Autodesk Inventor part; units mm, degrees
ref_plane "YZ Plane" through (0, 0, 0) normal (1, 0, 0) x (0, 1, 0)
ref_plane "XZ Plane" through (0, 0, 0) normal (0, 1, 0) x (-1, 0, 0)
ref_plane "XY Plane" through (0, 0, 0) normal (0, 0, 1) x (1, 0, 0)
sketch "スケッチ3" plane through (0, 0, 0) normal (0, 0, 1) x (1, 0, 0)
  line L0 (0, 0) -> (0, 5)
  line L1 (0, 5) -> (-10, 5)
  line L2 (-10, 5) -> (-20, 15)
  line L3 (-20, 15) -> (-35, 15)
  line L4 (-35, 15) -> (-45, 5)
  line L5 (-45, 5) -> (-55, 15)
  line L6 (-80, 0) -> (0, 0)
  line L7 (0, 5) -> (0, 0)
  line L8 (-55, 15) -> (-80, 15)
  line L9 (-80, 15) -> (-80, 0)
  dimension "d0" = 10
  dimension "d2" = 15
  dimension "d4" = 5
  dimension "d6" = 135
  dimension "d9" = 25
  dimension "d10" = 15
extrude "押し出し1" add sketch "スケッチ3" along normal blind 15
chamfer "面取り1" distance 4 angle 45 1 edges at (-80, 15, 7.5)
sketch "スケッチ4" plane through (0, 0, 15) normal (0, 0, 1) x (1, 0, 0)
  line L0 (-80, 11) -> (-76, 15)
  line L1 (-80, 11) -> (-80, 0)
  line L2 (-80, 0) -> (0, 0)
  line L3 (0, 0) -> (0, 5)
  line L4 (0, 5) -> (-10, 5)
  line L5 (-10, 5) -> (-20, 15)
  line L6 (-20, 15) -> (-35, 15)
  line L7 (-35, 15) -> (-45, 5)
  line L8 (-45, 5) -> (-55, 15)
  line L9 (-55, 15) -> (-76, 15)
  line L10 (-93.9194, 12.5) -> (6.2827, 12.5)
  line L11 (-45, 5) -> (-55, 15)
  line L12 (-35, 15) -> (-45, 5)
  line L13 (-10, 5) -> (-20, 15)
  line L14 (-65.5, 45.5) -> (-65.5, -30.5) construction
  line L15 (-55, 15) -> (-76, 15) construction
  line L16 (-55, 15) -> (-55, -16.6145) construction
  line L17 (-76, 15) -> (-76, -16.6145) construction
  point P0 (-78.5, 12.5)
  point P1 (-52.5, 12.5)
  point P2 (-37.5, 12.5)
  point P3 (-17.5, 12.5)
  dimension "d14" = 12.5
  dimension "d15" = 17.5
  dimension "d16" = 37.5
  dimension "d17" = 52.5
  dimension "d18" = 78.5
  dimension "d19" = 65.5
properties part number "finger2"
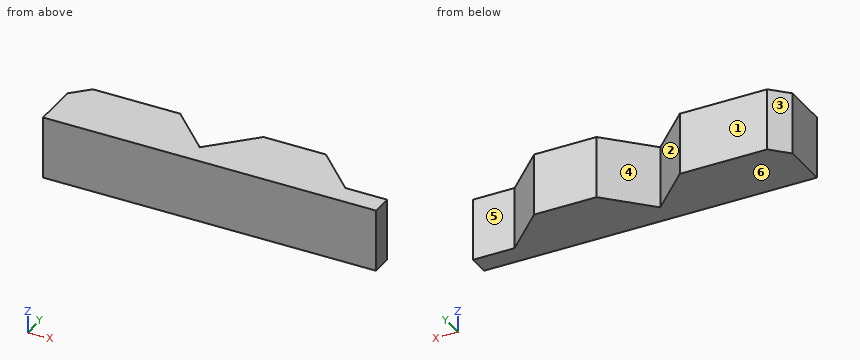
CAD build for the part. Positions are in the model's coordinates, mm. Face numbers are marked on the shaded views. A direction names the side the tool comes from. Coordinates: 2 decimals unless noted, no trailing zeros. Write each loop counter-clockwise with the first axis right and the second up, starting at its lowest first coordinate (ties: lowest second). Pieces come first, ordered by that corner, then holes. Notation, with made-up numbers: M 88.25,12.25 L 130.25,12.25 A6 cw 130.25,23.25 Z; hole C 16,38.25 d2. An arc over 180 degrees is marked long. Return JSON: item names as keys, results as strings.
Item 1: Drop flat-ended pins along their axis: pin 1 Ø4 at (y, z) = (9.5, 5.5) entering from +X; pin 2 Ø6 at (x, y) = (-42, 12) entering from -Z. Give the stop position or say it passes through.
Findings below:
{"pin 1": "stops at x = -12.5", "pin 2": "stops at z = 0"}
Item 2: Slice it at A-A, the plane y = 9.5. Write the cut outline in (x, z), and give its area (4 significant figures).
Findings below:
{"outline": "M -80,0 L -49.5,0 L -49.5,15 L -80,15 Z; M -40.5,0 L -14.5,0 L -14.5,15 L -40.5,15 Z", "area": "847.5 mm2"}
Item 3: Which spindle directions (+Z, -Z, +X, -X, +Y, -Y) get a long thin tool onto all of the face, cutting with end or side? Do the marked faces 4, 5 and 6. Say none if no direction does.
Findings below:
{"face 4": "+Z, -Z, +Y", "face 5": "+Z, -Z, +X, +Y", "face 6": "-Z, +X, -X, +Y, -Y"}
Item 4: Slice it at B-B, the plane z = 6.25. Write the cut outline in (x, y), and give its area (3 significant figures).
Findings below:
{"outline": "M -80,0 L 0,0 L 0,5 L -10,5 L -20,15 L -35,15 L -45,5 L -55,15 L -76,15 L -80,11 Z", "area": "942 mm2"}
Item 5: Two-plate mould, pull along X, no slides. Class the marked faces 1, 2 and 3: +X half, -X half, draft (parallel to the pull), parting line (faces both ways), or undercut.
Findings below:
{"face 1": "draft", "face 2": "undercut", "face 3": "-X half"}
Item 6: Probe line 1 (Y direction, x = -3.5, z = 9); line 2 (X direction, y = 13, z = 7.5); line 3 (X direction, y = 6.5, z = 13). List the from-to ranges inside material, lowest first. Write a range as from..to.
Findings below:
{"line 1": "y = 0..5", "line 2": "x = -78..-53, -37..-18", "line 3": "x = -80..-46.5, -43.5..-11.5"}
Item 7: Slice it at D-D, the plane x = -46.5. Write the cut outline in (y, z), and give its area (3 significant figures).
Findings below:
{"outline": "M 0,0 L 6.5,0 L 6.5,15 L 0,15 Z", "area": "97.5 mm2"}
Item 8: Slice it at C-C, the plane x = -37. Write the cut outline in (y, z), and give its area (3 significant figures).
Findings below:
{"outline": "M 0,0 L 13,0 L 13,15 L 0,15 Z", "area": "195 mm2"}
